Part model, mm, in its own coordinate system. Face numbers are marked on the shaded views. Round coordinates to 2 decimals unless told otherwise and drop trailing zeros. Loops run counter-clockwise (first coordinate to the right, second up) from the corner with the lowest first, then second, coordinate; pieces in that order, holes last.
1) Drop a flat-ended pin along its axis: P1, Ø3, axis at x = 4, y = -3, coming from the +Z side (3 decimals). Give the stop position or say it passes through.
2) Band-saw the part on A-A, the plane z = -6.15. Write the cut outline in (x, y) (3 decimals), then the cut area to 3 significant figures.
3) Probe line 1 (X direction, y = 0, z = -6.3) (3 decimals); line 2 (Y direction, x = 0, z = -6.2) (3 decimals). List the from-to ranges inside material, lowest first.
4) Mould opens along Y. For the marked faces 1, 2, 3 and 4 say: +Y half, -Y half, draft (parallel to the pull), parting line (faces both ways), or undercut.
5) Band-saw the part on B-B, the plane x = 0. Write the cut outline in (y, z) (3 decimals).
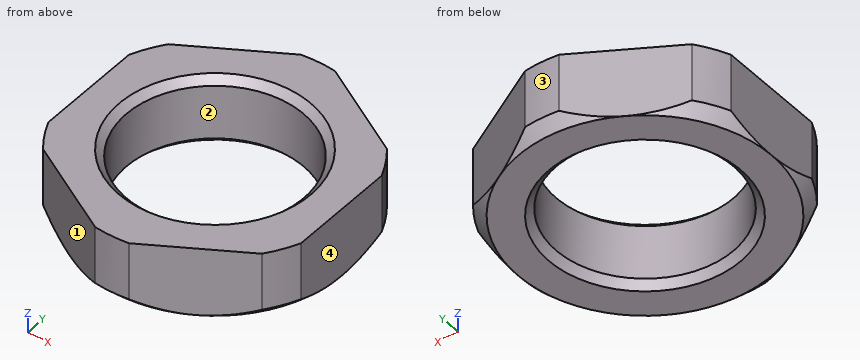
from build123d import *

# Parameters (mm, degrees)
SKETCH005_R     = 15.040905
POCKET002_DEPTH = 4.751
CHAMFER_SIZE    = 0.5


with BuildPart() as part:
    # Sketch004 → Revolution002 (revolve)
    with BuildSketch(Plane.YZ):
        Polygon((6.125, 0), (6.125, -4.75), (8.75, -4.75), (9.5, -4), (9.5, 0), align=None)
    revolve(axis=Axis((0, 0, 0), (0, 0, 1)))

    # Sketch005 (on Face2 of Revolution002) → Pocket002 (cut, through all)
    with BuildSketch(Plane.YX.offset(4.75)):
        Circle(SKETCH005_R)
        Polygon((10.10363, 0), (5.051815, 8.75), (-5.051815, 8.75), (-10.10363, 0), (-5.051815, -8.75), (5.051815, -8.75), align=None, mode=Mode.SUBTRACT)
    extrude(amount=-POCKET002_DEPTH, mode=Mode.SUBTRACT)

    # Chamfer
    chamfer_edges = [part.edges().sort_by_distance(p)[0] for p in [
        (0, -6.125, -4.75),
        (0, -6.125, 0),
    ]]
    chamfer(chamfer_edges, length=CHAMFER_SIZE)


with BuildPart() as part_1:
    # Body002 placement: moved
    add(part.part.moved(Location((0, 0, -2.9))))


solid = part_1.part
Reported:
1. P1: stops at z = -3.025
2. outline: (-8.75, -3.7) arc R9.5 ccw to (-7.579, -5.728) - (-1.171, -9.428) arc R9.5 ccw to (1.171, -9.428) - (7.579, -5.728) arc R9.5 ccw to (8.75, -3.7) - (8.75, 3.7) arc R9.5 ccw to (7.579, 5.728) - (1.171, 9.428) arc R9.5 ccw to (-1.171, 9.428) - (-7.579, 5.728) arc R9.5 ccw to (-8.75, 3.7) - close; hole circle Ø12.25 at (0, 0)
2. area: 143 mm2
3. line 1: x = -8.75 to -6.125, 6.125 to 8.75
3. line 2: y = -9.5 to -6.125, 6.125 to 9.5
4. face 1: -Y half
4. face 2: undercut
4. face 3: +Y half
4. face 4: draft
5. outline: (-9.5, -6.9) - (-8.75, -7.65) - (-6.625, -7.65) - (-6.125, -7.15) - (-6.125, -3.4) - (-6.625, -2.9) - (-9.5, -2.9) - close; (6.125, -7.15) - (6.625, -7.65) - (8.75, -7.65) - (9.5, -6.9) - (9.5, -2.9) - (6.625, -2.9) - (6.125, -3.4) - close
